```python
from build123d import *

# Parameters (mm, degrees)
SKETCH_1_R               = 12
SKETCH_1_R_2             = 8
EXTRUDE_1_DEPTH          = 4
CUT_EXTRUDE_1_DEPTH      = 19.761663039
CUT_EXTRUDE_1_DEPTH_BACK = 3
SKETCH_3_W               = 39.283858622
SKETCH_3_H               = 1.5


# Read off the part's stored shape, not the designer's step: M24 机械螺纹 螺柱1
with BuildPart() as part:
    # 草图1 → 凸台-拉伸1 (new, symmetric)
    with BuildSketch(Plane.XY):
        Circle(SKETCH_1_R)
        Circle(SKETCH_1_R_2, mode=Mode.SUBTRACT)
    extrude(amount=EXTRUDE_1_DEPTH, both=True)

    # M24 机械螺纹 螺柱1 outline → M24 机械螺纹 螺柱1 (revolve, cut)
    with BuildSketch(Plane.XZ):
        Polygon((12, 4), (10.376, 4), (12, 2.376), align=None)
    revolve(axis=Axis((0, 0, 0), (0, 0, 1)), mode=Mode.SUBTRACT)

    # 草图3 → 切除-拉伸-薄壁1 (cut, two sides: drawn at the far end of the back side and taken through both)
    with BuildSketch(Plane(origin=(0, 0, -4), x_dir=(-1, 0, 0), z_dir=(0, 0, -1)).offset(-CUT_EXTRUDE_1_DEPTH_BACK)):
        Rectangle(SKETCH_3_W, SKETCH_3_H)
    extrude(amount=CUT_EXTRUDE_1_DEPTH + CUT_EXTRUDE_1_DEPTH_BACK, mode=Mode.SUBTRACT)


solid = part.part
```
Could you check a few things on this model? Use its own coordinates, in mm. A direction names the side the tool comes from. Round coordinates to 2 decimals unless told otherwise and drop trailing zeros. Loops run counter-clockwise (first coordinate to the right, second up) from the corner with the lowest first, then second, coordinate; pieces in that order, holes last. Notation, with made-up numbers: (-24.5, 40.5) - (28.5, 40.5) arc R36 cw to (28.5, 78.5) - close; hole circle Ø4 at (15.25, -38). An arc over 180 degrees is marked (long way). Answer in a Markdown table with one row per item. Add a question column.
(1) I need wall thicknesses on line 1 along Y through (x, z) = (0, 2); line 2 along X through (y, z) = (2.75, 0.5). Which ranges of each line are inside material? Lowest first, please.
(2) If we section it at D-D (z = 3.5): Please give me the cut outline in (x, y).
(3) If we mould it in two halves opening along Y, with no side actions, what happens to faces 3 (the face through (11.446, 3.604, -0.767)), 4 (the face through (0, 9, -4)), 5 (the face through (10, 0, -1))? For each: pulls with the +Y half, pulls with the -Y half, needs draft (parallel to the pull), parting line crosses it, or undercut.
(4) For faces 1 (the face through (7.39, -3.06, -0.06)), 2 (the face through (10, -0.75, -2)), which set-ups out of +Z, -Z, +X, -X, +Y, -Y let a thin tool reach every point of the face, with its end or its side?
(5) I'm going to push flat-ended pins straight in: pin 1 (1.5 mm diameter, centred on x = 8.5, y = 9, fed in from +Z); pin 2 (0.8 mm diameter, centred on x = 9.5, y = 0, fed in from -Z); pin 3 (2.5 mm diameter, centred on x = 10, z = -3, fed in from +Y). Where does each tip first touch, or does it pass through?
(6) If we section it at B-B (y = 0): Please give me the cut outline in (x, z), plus the area to 3 significant figures.
(7) If we section it at C-C (x = 0): Please give me the cut outline in (y, z), plus the area to 3 significant figures.
Model answer:
| question | item | result |
|---|---|---|
| 1 | line 1 | y = -12 to -8, 8 to 12 |
| 1 | line 2 | x = -11.68 to -7.51, 7.51 to 11.68 |
| 2 | outline | circle Ø21.75 at (0, 0); hole circle Ø16 at (0, 0) |
| 3 | face 3 | parting line crosses it |
| 3 | face 4 | needs draft |
| 3 | face 5 | undercut |
| 4 | face 1 | +Z, -Z |
| 4 | face 2 | -Z, +X, -X |
| 5 | pin 1 | stops at z = 2.75 |
| 5 | pin 2 | stops at z = -1 |
| 5 | pin 3 | stops at y = 8.21 |
| 6 | outline | (-12, -1) - (-8, -1) - (-8, 4) - (-10.38, 4) - (-12, 2.38) - close; (8, -1) - (12, -1) - (12, 2.38) - (10.38, 4) - (8, 4) - close |
| 6 | area | 37.4 mm² |
| 7 | outline | (-12, -4) - (-8, -4) - (-8, 4) - (-10.38, 4) - (-12, 2.38) - close; (8, -4) - (12, -4) - (12, 2.38) - (10.38, 4) - (8, 4) - close |
| 7 | area | 61.4 mm² |
